Autodesk Inventor part; units mm, degrees
ref_plane "YZ Plane" through (0, 0, 0) normal (1, 0, 0) x (0, 1, 0)
ref_plane "XZ Plane" through (0, 0, 0) normal (0, 1, 0) x (-1, 0, 0)
ref_plane "XY Plane" through (0, 0, 0) normal (0, 0, 1) x (1, 0, 0)
sketch "Sketch1" plane through (0, 0, 0) normal (0, 1, 0) x (-1, 0, 0)
  line L0 (0, 0) -> (10, 0)
  line L1 (10, 0) -> (10, -3.5)
  line L2 (10, -3.5) -> (0, -3.5)
  line L3 (0, -3.5) -> (0, 0)
  line L4 (10, -3.5) -> (0, -3.5)
  line L5 (0, -3.5) -> (0, -6)
  line L6 (0, -6) -> (10, -6)
  line L7 (10, -6) -> (10, -3.5)
  line L8 (10, -6) -> (0, -6)
  line L9 (0, -6) -> (0, -9.5)
  line L10 (0, -9.5) -> (10, -9.5)
  line L11 (10, -9.5) -> (10, -6)
  line L12 (10, -9.5) -> (0, -9.5)
  line L13 (0, -9.5) -> (0, -12)
  line L14 (0, -12) -> (10, -12)
  line L15 (10, -12) -> (10, -9.5)
  line L16 (10, -12) -> (0, -12)
  line L17 (0, -12) -> (0, -15.5)
  line L18 (0, -15.5) -> (10, -15.5)
  line L19 (10, -15.5) -> (10, -12)
  line L20 (10, -7.75) -> (5, -7.75)
  circle A0 centre (5, -7.75) radius 1.5
  dimension "d0" = 10
  dimension "d1" = 3.5
  dimension "d2" = 2.5
  dimension "d3" = 10
  dimension "d4" = 3.5
  dimension "d5" = 10
  dimension "d6" = 2.5
  dimension "d7" = 3.5
  dimension "d12" = 5
  dimension "d13" = 3
extrude "Extrusion1" add sketch "Sketch1" against normal blind 2
extrude "Extrusion2" add sketch "Sketch1" along normal blind 2.4 contours L0 L1 L2 L3 | L14 L19 L18 L17
extrude "Extrusion3" add sketch "Sketch1" along normal blind 2.2 contours L6 L11 L10 L9
properties part number "yellow_plate_screw_grip_1"
For this review, take the finished solid that the model builds, in its own axes (mm). A direction names the side the tool comes from. Coordinates: 2 decimals unless noted, no trailing zeros. Loops run counter-clockwise (first coordinate to the right, second up) from the corner with the lowest first, then second, coordinate; pieces in that order, holes last. Notation, with made-up numbers: (60, -5) -> (105, -5) arc R10 ccw to (105, 7) -> close; hole circle Ø7 at (14, -14.75). An arc over 180 degrees is marked (long way). Return JSON: item names as keys, results as strings. Group by question number.
(1) Consider section A-A, the plane y = 1.85. Give the boundary of the cut face in (x, z).
(2) To check wall thickness, follow L1, parallel to Z at x = -8.25, y = 1.15; L2, parallel to Z at x = -5, y = 1; L3, parallel to Z at x = -6.75, y = 2.25. State the ranges of each line that lie inside material, in increasing order.
(3) Consider section D-D, the plane x = -1.5. Give the boundary of the cut face in (y, z), plus the area to 3 significant figures.
(4) Tool access review of faces 1 (the flat face through (-3.8, 2.2, -6.6)), 2 (the flat face through (-5, 2.4, -2)): name each direction out of +Z, -Z, +X, -X, +Y, -Y from which nothing blocks a thin tool from reaching the whole face with its end or side.
(5) Consider section C-C, the plane z = -7.75. Give the boundary of the cut face in (x, y).
(6) For pin 1 Ø4 at (x, z) = (-3, -8.5) entering from +Y; pin 2 Ø1.2 at (x, z) = (-7, -4.5) entering from +Y, all flat-tipped, find the tip position at first contact; note any pin that passes through.
(7) Mouldability with a two-part tool opening along Z and no side actions: class faces 3 (the flat face through (-5, 1, -9.5)), 4 (the flat face through (-4.9, -2, -9.4)), 5 (the flat face through (-5, 0, -15.5)) as pulls with the +Z half, pulls with the -Z half, needs draft (parallel to the pull), parting line crosses it, or undercut.
(8) Consider section B-B, the plane x = -5. Give the boundary of the cut face in (y, z).
Results below:
{
 "1": {"outline": "(-10, -15.5) -> (0, -15.5) -> (0, -12) -> (-10, -12) -> close; (-10, -9.5) -> (0, -9.5) -> (0, -6) -> (-10, -6) -> close; (-10, -3.5) -> (0, -3.5) -> (0, 0) -> (-10, 0) -> close; hole circle Ø3 at (-5, -7.75)"},
 "2": {"L1": "z = -15.5 to -12, -9.5 to -6, -3.5 to 0", "L2": "z = -15.5 to -12, -9.5 to -9.25, -6.25 to -6, -3.5 to 0", "L3": "z = -15.5 to -12, -3.5 to 0"},
 "3": {"outline": "(-2, -15.5) -> (2.4, -15.5) -> (2.4, -12) -> (0, -12) -> (0, -9.5) -> (2.2, -9.5) -> (2.2, -6) -> (0, -6) -> (0, -3.5) -> (2.4, -3.5) -> (2.4, 0) -> (-2, 0) -> close", "area": "55.5 mm2"},
 "4": {"face 1": "+X, -X, +Y", "face 2": "+Z, -Z, +X, -X, +Y"},
 "5": {"outline": "(-10, -2) -> (-6.5, -2) -> (-6.5, 2.2) -> (-10, 2.2) -> close; (-3.5, -2) -> (0, -2) -> (0, 2.2) -> (-3.5, 2.2) -> close"},
 "6": {"pin 1": "stops at y = 2.2", "pin 2": "stops at y = 0"},
 "7": {"face 3": "undercut", "face 4": "needs draft", "face 5": "pulls with the -Z half"},
 "8": {"outline": "(-2, -15.5) -> (2.4, -15.5) -> (2.4, -12) -> (0, -12) -> (0, -9.5) -> (2.2, -9.5) -> (2.2, -9.25) -> (-2, -9.25) -> close; (-2, -6.25) -> (2.2, -6.25) -> (2.2, -6) -> (0, -6) -> (0, -3.5) -> (2.4, -3.5) -> (2.4, 0) -> (-2, 0) -> close"}
}
